```python
from build123d import *

# Parameters (mm, degrees)
SKETCH1_R           = 30
BOSS_EXTRUDE1_DEPTH = 15
SKETCH2_R           = 10
BOSS_EXTRUDE2_DEPTH = 103
SKETCH4_R           = 7.25
CUT_EXTRUDE1_DEPTH  = 57
SKETCH5_R           = 5
CUT_EXTRUDE2_DEPTH  = 62
SKETCH7_R           = 6.5
CUT_EXTRUDE3_DEPTH  = 6.6
SKETCH8_R           = 3.2
CUT_EXTRUDE4_DEPTH  = 9.4
CIRPATTERN1_COUNT   = 4


with BuildPart() as part:
    # Sketch1 → Boss-Extrude1 (new body)
    with BuildSketch(Plane(origin=(0, 0, 0), x_dir=(1, 0, 0), z_dir=(0, 1, 0))):
        Circle(SKETCH1_R)
    extrude(amount=BOSS_EXTRUDE1_DEPTH)

    # Sketch2 → Boss-Extrude2 (add)
    with BuildSketch(Plane(origin=(0, 15, 0), x_dir=(1, 0, 0), z_dir=(0, 1, 0))):
        Circle(SKETCH2_R)
    extrude(amount=BOSS_EXTRUDE2_DEPTH)

    # Sketch4 → Cut-Extrude1 (cut)
    with BuildSketch(Plane.XZ):
        Circle(SKETCH4_R)
    extrude(amount=-CUT_EXTRUDE1_DEPTH, mode=Mode.SUBTRACT)

    # Sketch5 → Cut-Extrude2 (cut, through all)
    with BuildSketch(Plane.XZ.offset(-57)):
        Circle(SKETCH5_R)
    extrude(amount=-CUT_EXTRUDE2_DEPTH, mode=Mode.SUBTRACT)

    # Sketch7 → Cut-Extrude3 (cut)
    with BuildSketch(Plane(origin=(0, 15, 0), x_dir=(1, 0, 0), z_dir=(0, 1, 0))):
        with Locations((0, -20)):
            Circle(SKETCH7_R)
    cut_extrude3 = extrude(amount=-CUT_EXTRUDE3_DEPTH, mode=Mode.SUBTRACT)

    # Sketch8 → Cut-Extrude4 (cut, through all)
    with BuildSketch(Plane(origin=(0, 8.4, 0), x_dir=(1, 0, 0), z_dir=(0, 1, 0))):
        with Locations((0, -20)):
            Circle(SKETCH8_R)
    cut_extrude4 = extrude(amount=-CUT_EXTRUDE4_DEPTH, mode=Mode.SUBTRACT)

    # CirPattern1: Cut-Extrude3, Cut-Extrude4 ×4 about axis
    cirpattern1_axis = Axis((0, 0, 0), (0, 1, 0))
    for i in range(1, CIRPATTERN1_COUNT):
        add(cut_extrude3.rotate(cirpattern1_axis, i * 360 / CIRPATTERN1_COUNT), mode=Mode.SUBTRACT)
        add(cut_extrude4.rotate(cirpattern1_axis, i * 360 / CIRPATTERN1_COUNT), mode=Mode.SUBTRACT)


solid = part.part
```
Could you check a few things on this model? Use its own coordinates, in mm. A direction names the side the tool comes from. Give positions to 0.01 mm unless a question says otherwise; leave off trailing zeros. Loops run counter-clockwise (first coordinate to the right, second up) from the corner with the lowest first, then second, coordinate; pieces in that order, holes last. Notation, with made-up numbers: (-40, -1) -> (15, -1) arc R24 ccw to (15, 14) -> close; hole circle Ø6 at (-33, 89). An arc over 180 degrees is marked (long way). Put each result on its own line as item: value.
(1) I'm going to push flat-ended pins straight in: pin 1 Ø13 at (x, z) = (0, 0) entering from -Y; pin 2 Ø10 at (y, z) = (98.5, 5.5) entering from +X; pin 3 Ø14.5 at (x, z) = (2.5, 22) entering from +Y. Where does each tip first touch, or does it pass through?
Computed:
pin 1: y = 57
pin 2: x = 9.99
pin 3: y = 15
(2) Imagine slicing it at A-A on x = 0. State how many separate pieces and enclosed holes the cut face has, plus the area to 3 significant figures.
Computed:
separate pieces: 4
enclosed holes: 0
area: 1,240 mm^2
(3) For faces 4 (the face through (-1.08, 87.07, -4.88)), 5 (the face through (-2, 57, -5)), 6 (the face through (17, 8.4, 2)), which set-ups out of +Z, -Z, +X, -X, +Y, -Y let a thin tool reach every point of the face, with its end or its side?
Computed:
face 4: +Y, -Y
face 5: -Y
face 6: +Y
(4) Imagine slicing it at C-C on x = 21.5. Write out the boundary of the cut face in (y, z).
Computed:
outline: (0, -20.92) -> (15, -20.92) -> (15, -6.32) -> (8.4, -6.32) -> (8.4, -2.83) -> (0, -2.83) -> close; (0, 2.83) -> (8.4, 2.83) -> (8.4, 6.32) -> (15, 6.32) -> (15, 20.92) -> (0, 20.92) -> close
(5) Imagine slicing it at D-D on z = 20. Write out the boundary of the cut face in (x, y).
Computed:
outline: (-22.36, 0) -> (-3.2, 0) -> (-3.2, 8.4) -> (-6.5, 8.4) -> (-6.5, 15) -> (-22.36, 15) -> close; (3.2, 0) -> (22.36, 0) -> (22.36, 15) -> (6.5, 15) -> (6.5, 8.4) -> (3.2, 8.4) -> close
(6) Please list where these lines run through material, in increasing order: probe 1 along Z at (x, y) = (0, 11.25); probe 2 along Z at (x, y) = (0, 5.5); probe 3 along Z at (x, y) = (0, 102). Write a range as [from, to].
Computed:
probe 1: [-30, -26.5], [-13.5, -7.25], [7.25, 13.5], [26.5, 30]
probe 2: [-30, -23.2], [-16.8, -7.25], [7.25, 16.8], [23.2, 30]
probe 3: [-10, -5], [5, 10]
(7) Thinking about a two-plate mould opening in Z: for faces 1 (the face through (-29.97, 7.4, -1.32)), 2 (the face through (13, 15, 0)), 3 (the face through (-23.124, 4.259, -0.694)), which applies, pulls with the +Z half, pulls with the -Z half, needs draft (parallel to the pull), parting line crosses it, or undercut?
Computed:
face 1: parting line crosses it
face 2: needs draft
face 3: undercut
